Geometry check sheet. Reference: the model listing, model coordinates, mm. A direction names the side the tool comes from. Round coordinates to 2 decimals unless told otherwise and drop trailing zeros. Loops run counter-clockwise (first coordinate to the right, second up) from the corner with the lowest first, then second, coordinate; pieces in that order, holes last. Notation, with made-up numbers: M -24.75,-1 L -3.75,-1 A13 ccw -3.75,7 Z; hole C -15.75,23.25 d4. An arc over 180 degrees is marked long. Answer in a Markdown table with one row per item. Add a question column.
```python
from build123d import *

# Parameters (mm, degrees)
SKETCH_1_W          = 160
SKETCH_1_H          = 120
EXTRUDE_1_DEPTH     = 30
CUT_EXTRUDE_1_DEPTH = 31
CHAMFER_1_SIZE      = 10
SKETCH_3_R          = 15
CUT_EXTRUDE_2_DEPTH = 30


with BuildPart() as part:
    # 草图1 → 凸台-拉伸1 (new body)
    with BuildSketch(Plane.XY):
        Rectangle(SKETCH_1_W, SKETCH_1_H)
    extrude(amount=EXTRUDE_1_DEPTH)

    # 草图2 → 切除-拉伸1 (cut, through all)
    with BuildSketch(Plane.XY.offset(30)):
        with BuildLine():
            Line((-65, 34.5), (-35, 34.5))
            ThreePointArc((-35, 34.5), (-30.5, 30), (-35, 25.5))
            Line((-35, 25.5), (-65, 25.5))
            ThreePointArc((-65, 25.5), (-69.5, 30), (-65, 34.5))
        make_face()
        with BuildLine():
            Line((65, 25.5), (35, 25.5))
            ThreePointArc((35, 25.5), (30.5, 30), (35, 34.5))
            Line((35, 34.5), (65, 34.5))
            ThreePointArc((65, 34.5), (69.5, 30), (65, 25.5))
        make_face()
        with BuildLine():
            Line((-65, -25.5), (-35, -25.5))
            ThreePointArc((-35, -25.5), (-30.5, -30), (-35, -34.5))
            Line((-35, -34.5), (-65, -34.5))
            ThreePointArc((-65, -34.5), (-69.5, -30), (-65, -25.5))
        make_face()
        with BuildLine():
            Line((65, -34.5), (35, -34.5))
            ThreePointArc((35, -34.5), (30.5, -30), (35, -25.5))
            Line((35, -25.5), (65, -25.5))
            ThreePointArc((65, -25.5), (69.5, -30), (65, -34.5))
        make_face()
    extrude(amount=-CUT_EXTRUDE_1_DEPTH, mode=Mode.SUBTRACT)

    # 倒角1
    chamfer_1_edges = [part.edges().sort_by_distance(p)[0] for p in [
        (-80, 60, 15),
        (80, 60, 15),
        (80, -60, 15),
        (-80, -60, 15),
    ]]
    chamfer(chamfer_1_edges, length=CHAMFER_1_SIZE)

    # 草图3 → 切除-拉伸2 (cut)
    with BuildSketch(Plane.XY.offset(30)):
        Circle(SKETCH_3_R)
    extrude(amount=-CUT_EXTRUDE_2_DEPTH, mode=Mode.SUBTRACT)


solid = part.part
```
1) Set-up check for faces 1 (the cylindrical face through (30.5, 29.9, 15.2)), 2 (the flat face through (75, 55, 15)): record each of +Z, -Z, +X, -X, +Y, -Y from which the full face is reachable in a straight line by a thin tool's end or side.
2) Cross-section at D-D, the plane x = -45.5. Record the boundary of the cut face in (y, z).
3) Cross-section at A-A, the plane z = 19.5. Record the boundary of the cut face in (x, y).
4) Draft check along X on faces 3 (the flat face through (-1, -60, 15)), 4 (the flat face through (-75, -55, 15)), 5 (the cylindrical face through (-69.5, 29.9, 15.2)). Enter one of: +X half, -X half, draft (parallel to the pull), parting line (faces both ways), or undercut.
5) Thickness scan on L1, parallel to Y at x = 65.5, z = 8.25; L2, parallel to X at y = -32, z = 4; L3, parallel to Y at x = 0, z = 22.25. Record the ranges inside material, lowest first. Write a range as [from, to].
6) Cross-section at B-B, the plane x = 0. Record the boundary of the cut face in (y, z), plus the area to 3 significant figures.
7) Cross-section at C-C, the plane y = -30. Record the boundary of the cut face in (x, z).
Worked answers:
| question | item | result |
|---|---|---|
| 1 | face 1 | +Z, -Z |
| 1 | face 2 | +Z, -Z, +X, +Y |
| 2 | outline | M -60,0 L -34.5,0 L -34.5,30 L -60,30 Z; M -25.5,0 L 25.5,0 L 25.5,30 L -25.5,30 Z; M 34.5,0 L 60,0 L 60,30 L 34.5,30 Z |
| 3 | outline | M -80,-50 L -70,-60 L 70,-60 L 80,-50 L 80,50 L 70,60 L -70,60 L -80,50 Z; hole M -65,-34.5 L -35,-34.5 A4.5 ccw -35,-25.5 L -65,-25.5 A4.5 ccw Z; hole M -65,25.5 L -35,25.5 A4.5 ccw -35,34.5 L -65,34.5 A4.5 ccw Z; hole C 0,0 d30; hole M 35,-34.5 L 65,-34.5 A4.5 ccw 65,-25.5 L 35,-25.5 A4.5 ccw Z; hole M 35,25.5 L 65,25.5 A4.5 ccw 65,34.5 L 35,34.5 A4.5 ccw Z |
| 4 | face 3 | draft |
| 4 | face 4 | -X half |
| 4 | face 5 | undercut |
| 5 | L1 | y = [-60, -34.47], [-25.53, 25.53], [34.47, 60] |
| 5 | L2 | x = [-80, -69.03], [-30.97, 30.97], [69.03, 80] |
| 5 | L3 | y = [-60, -15], [15, 60] |
| 6 | outline | M -60,0 L -15,0 L -15,30 L -60,30 Z; M 15,0 L 60,0 L 60,30 L 15,30 Z |
| 6 | area | 2,700 mm2 |
| 7 | outline | M -80,0 L -69.5,0 L -69.5,30 L -80,30 Z; M -30.5,0 L 30.5,0 L 30.5,30 L -30.5,30 Z; M 69.5,0 L 80,0 L 80,30 L 69.5,30 Z |
